Work out the finished part from the listing and answer in its coordinate system (mm). A direction names the side the tool comes from. Round coordinates to 2 decimals unless told otherwise and drop trailing zeros. Loops run counter-clockwise (first coordinate to the right, second up) from the corner with the lowest first, then second, coordinate; pieces in that order, holes last. Notation, with made-up numbers: (-19.75, 52) - (30.25, 52) arc R17 ccw to (30.25, 79) - close; hole circle Ø7 at (28.25, 81). An arc over 180 degrees is marked (long way). Return JSON: item names as keys, results as strings.
from build123d import *

# Parameters (mm, degrees)
F0_R     = 7
F0_R_2   = 4.7
F0_R_3   = 3
F1_DEPTH = 2
F2_DEPTH = 12
F0_R_4   = 4.65
F3_DEPTH = 2
F0_R_5   = 3.05
F4_DEPTH = 12
F0_W     = 31.71593739
F0_H     = 26.2385108796
F5_DEPTH = 0.3


with BuildPart() as f1:
    # F0 (on Top) → F1 (new body)
    with BuildSketch(Plane.XY):
        Circle(F0_R)
        Circle(F0_R_2, mode=Mode.SUBTRACT)
        Circle(F0_R_2)
        Circle(F0_R_3, mode=Mode.SUBTRACT)
    extrude(amount=F1_DEPTH)

    # F0 (on Top) → F2 (join)
    with BuildSketch(Plane.XY):
        Circle(F0_R_2)
        Circle(F0_R_3, mode=Mode.SUBTRACT)
    extrude(amount=F2_DEPTH)



with BuildPart() as f3:
    # F0 (on Top) → F3 (new body)
    with BuildSketch(Plane.XY):
        with Locations((-13.71593739, -8.2385108796)):
            Circle(F0_R)
        with Locations((-13.71593739, -8.2385108796)):
            Circle(F0_R_4, mode=Mode.SUBTRACT)
    extrude(amount=F3_DEPTH)

    # F0 (on Top) → F4 (join)
    with BuildSketch(Plane.XY):
        with Locations((-13.71593739, -8.2385108796)):
            Circle(F0_R_4)
        with Locations((-13.71593739, -8.2385108796)):
            Circle(F0_R_5, mode=Mode.SUBTRACT)
    extrude(amount=F4_DEPTH)


with BuildPart() as f1_1:
    add(f1.part)

    add(f3.part)  # F5 merges F3
    # F0 (on Top) → F5 (join)
    with BuildSketch(Plane.XY):
        with Locations((-6.857968695, -4.1192554398)):
            Rectangle(F0_W, F0_H)
        with Locations((-13.71593739, -8.2385108796)):
            Circle(F0_R, mode=Mode.SUBTRACT)
        Circle(F0_R, mode=Mode.SUBTRACT)
        with Locations((-13.71593739, -8.2385108796)):
            Circle(F0_R)
        with Locations((-13.71593739, -8.2385108796)):
            Circle(F0_R_4, mode=Mode.SUBTRACT)
        Circle(F0_R)
        Circle(F0_R_2, mode=Mode.SUBTRACT)
        Circle(F0_R_2)
        Circle(F0_R_3, mode=Mode.SUBTRACT)
        with Locations((-13.71593739, -8.2385108796)):
            Circle(F0_R_4)
        with Locations((-13.71593739, -8.2385108796)):
            Circle(F0_R_5, mode=Mode.SUBTRACT)
        with Locations((-13.71593739, -8.2385108796)):
            Circle(F0_R_5)
        Circle(F0_R_3)
    extrude(amount=F5_DEPTH)


solid = f1_1.part
1) Flat-ended cylindrical pins translate along their axes: pin 1 (6 mm diameter, centred on y = -4, z = 8.5, fed in from -X); pin 2 (4 mm diameter, centred on y = -9.5, z = 7.5, fed in from +X); pin 3 (2 mm diameter, centred on x = -3.5, z = 7, fed in from +Y). Find the tip coordinate at first contact, or state that the pin passes through.
Verdict:
{"pin 1": "stops at x = -18.2", "pin 2": "stops at x = -9.07", "pin 3": "stops at y = 3.98"}
2) A tool of negligible diameter and unlimited length cuts with its end or side. For faces 5 (the cylindrical face through (-3, 0, 6)), 6 (the flat face through (-12.7, -11.3, 12)), from which of +Z, -Z, +X, -X, +Y, -Y can it reach the whole face along a straight path? Write none if from no direction.
Verdict:
{"face 5": "+Z", "face 6": "+Z, +X, -X, +Y, -Y"}
3) Section B-B (y = 0) is taken. Give the vertices of the cut face in (x, z).
Verdict:
{"outline": "(-22.72, 0) - (9, 0) - (9, 0.3) - (7, 0.3) - (7, 2) - (4.7, 2) - (4.7, 12) - (3, 12) - (3, 0.3) - (-3, 0.3) - (-3, 12) - (-4.7, 12) - (-4.7, 2) - (-7, 2) - (-7, 0.3) - (-22.72, 0.3) - close"}
4) Find the intervals of material crossed by L1, parallel to Y at x = 0, z = 7.5; L2, parallel to Z at x = -12.5, y = -2.75; L3, parallel to Z at x = 3.5, y = -15.75, in increasing order.
Verdict:
{"L1": "y = -4.7 to -3, 3 to 4.7", "L2": "z = 0 to 2", "L3": "z = 0 to 0.3"}
5) Section D-D (y = -14.75) is taken. Give the vertices of the cut face in (x, z), and give its area (3 significant figures).
Verdict:
{"outline": "(-22.72, 0) - (9, 0) - (9, 0.3) - (-11.15, 0.3) - (-11.15, 2) - (-16.29, 2) - (-16.29, 0.3) - (-22.72, 0.3) - close", "area": "18.2 mm2"}
6) Determine the mould class of faces 1 (the cylindrical face through (-9.42, -10.02, 6.93)), 2 (the flat face through (1, -3, 12)), 3 (the cylindrical face through (-14.377, -11.216, 6.068)), 4 (the flat face through (-14, -8, 0.3)) for opening direction Y: pulls with the +Y half, pulls with the -Y half, needs draft (parallel to the pull), parting line crosses it, or undercut.
Verdict:
{"face 1": "parting line crosses it", "face 2": "needs draft", "face 3": "undercut", "face 4": "undercut"}
7) Section A-A (x = 0) is taken. Give the vertices of the cut face in (y, z), and give its area (3 significant figures).
Verdict:
{"outline": "(-17.24, 0) - (9, 0) - (9, 0.3) - (7, 0.3) - (7, 2) - (4.7, 2) - (4.7, 12) - (3, 12) - (3, 0.3) - (-3, 0.3) - (-3, 12) - (-4.7, 12) - (-4.7, 2) - (-7, 2) - (-7, 0.3) - (-17.24, 0.3) - close", "area": "55.5 mm2"}
8) Section C-C (z = 10.25) is taken. Give the vertices of the cut face in (x, y).
Verdict:
{"outline": "circle Ø9.3 at (-13.72, -8.24); circle Ø9.4 at (0, 0); hole circle Ø6.1 at (-13.72, -8.24); hole circle Ø6 at (0, 0)"}
